Source: CAD feature listing. Evaluate the final solid. Frame: model axes, mm. A direction names the side the tool comes from. Round coordinates to 2 decimals unless told otherwise and drop trailing zeros. Loops run counter-clockwise (first coordinate to the right, second up) from the corner with the lowest first, then second, coordinate; pieces in that order, holes last.
Item 1: Access query for faces 5 (the flat face through (-18, 54.636, 13)), 6 (the cylindrical face through (-13.866, 9.46, 30.61)), 7 (the flat face through (-7, -33.534, 37)), 8 (the cylindrical face through (-19.275, 56.525, 38.298)). Directions: +Z, -Z, +X, -X, +Y, -Y. A direction counts if a zero-diameter tool reaches every point of the face in a straight line with its end or side. Return the directions, or none.
Item 2: Section query C-C on x = 0. Give the number of separate pieces and of enclosed holes in the cut face, then the cut area to 3 significant figures.
Item 3: First-contact query: P1, Ø8, axis at x = 31, z = 0, coming from the -Y side; P2, Ø1.2, axis at y = 72, z = 29.5, coming from the -X side; P3, Ø6, axis at x = -9, z = -20, coming from the -Y side; P4, Ø8, axis at x = -40, z = 63.97, coming from the +Y side. Flat tips, straight axial feed; report the tip coordinate or a pass-through.
Item 4: Ray query, L1, parallel to Z at x = -15, y = 20.5; L2, parallel to Y at x = 14, z = -9.5; L3, parallel to Y at x = -8, z = 33.5. Return the intervals inside material, ascending.
Item 5: Pull-direction query (Y, two-part tool) for faces 1 (the cylindrical face through (-53.16, -20.17, -12.46)), 2 (the cylindrical face through (-42.44, 117.75, -39.52)), 3 (the cylindrical face through (-13.866, 9.46, -5.616)), 4 (the cylindrical face through (-13.866, 9.46, -15.904)); classes: released by +Y, released by -Y, zero draft, split by the parting line, or undercut.
Item 6: Section query B-B on x = -55. Return loops of the section in (y, z), then the cut area to 3 significant figures.
```python
from build123d import *

# Parameters (mm, degrees)
SKETCH1_R                = 45
BOSS_EXTRUDE1_DEPTH      = 25
BOSS_EXTRUDE2_DEPTH      = 25
BOSS_EXTRUDE2_DEPTH_BACK = 60
SKETCH3_R                = 16.694420179
BOSS_EXTRUDE3_DEPTH      = 10
SKETCH4_W                = 70
SKETCH4_H                = 114.66
BOSS_EXTRUDE4_DEPTH      = 5
SKETCH5_R                = 16.667292011
BOSS_EXTRUDE5_DEPTH      = 14
BOSS_EXTRUDE5_DEPTH_BACK = 39
FILLET1_R                = 10
FILLET2_R                = 40
FILLET3_R                = 20
FILLET4_R                = 5
FILLET5_R                = 2
SCALE1_SCALE             = 1.111111111
SKETCH6_W                = 73.333333333
SKETCH6_H                = 122.955555555
BOSS_EXTRUDE6_DEPTH      = 90
SKETCH7_R                = 2.5
CUT_EXTRUDE1_DEPTH       = 239.92789275
CUT_EXTRUDE1_DEPTH_BACK  = 239.92789275


with BuildPart() as part:
    # Sketch1 → Boss-Extrude1 (new body)
    with BuildSketch(Plane.XY):
        Circle(SKETCH1_R)
    extrude(amount=BOSS_EXTRUDE1_DEPTH)



with BuildPart() as body_2:
    # Sketch2 → Boss-Extrude2 (new, two sides)
    with BuildSketch(Plane(origin=(0, 0, 0), x_dir=(0, 0, -1), z_dir=(1, 0, 0))) as boss_extrude2_sk:
        Polygon((-32.711176171, -28.552814356), (-32.711176171, 50.79995961), (7.711176171, 50.79995961), (7.711176171, -28.552814356), (12.147045523, -28.552814356), (12.147045523, 54.003643031), (-37.147045523, 54.003643031), (-37.147045523, -28.552814356), align=None)
    extrude(amount=BOSS_EXTRUDE2_DEPTH)
    extrude(boss_extrude2_sk.sketch, amount=-BOSS_EXTRUDE2_DEPTH_BACK)

    # Sketch3 → Boss-Extrude3 (add)
    with BuildSketch(Plane(origin=(0, 54.003643031, 0), x_dir=(1, 0, 0), z_dir=(0, 1, 0))):
        with Locations(Location((-20, -13.418920015, 0), (0, 0, 270))):
            Circle(SKETCH3_R)
    extrude(amount=BOSS_EXTRUDE3_DEPTH)

    # Sketch4 → Boss-Extrude4 (add)
    with BuildSketch(Plane(origin=(0, 64.003643031, 0), x_dir=(1, 0, 0), z_dir=(0, 1, 0))):
        with Locations((-20, -12.5)):
            Rectangle(SKETCH4_W, SKETCH4_H)
    extrude(amount=BOSS_EXTRUDE4_DEPTH)


with BuildPart() as part_1:
    add(part.part)

    add(body_2.part)  # Boss-Extrude5 merges body 2
    # Sketch5 → Boss-Extrude5 (add, two sides)
    with BuildSketch(Plane(origin=(0, 0, 0), x_dir=(-1, 0, 0), z_dir=(0, 0, -1))) as boss_extrude5_sk:
        with Locations(Location((0, 0, 0), (0, 0, 180))):
            Circle(SKETCH5_R)
    extrude(amount=BOSS_EXTRUDE5_DEPTH)
    extrude(boss_extrude5_sk.sketch, amount=-BOSS_EXTRUDE5_DEPTH_BACK)

    # Fillet1
    fillet1_edges = [part_1.edges().sort_by_distance(p)[0] for p in [
        (-45, 0, 0),
        (-45, 0, 25),
    ]]
    fillet(fillet1_edges, radius=FILLET1_R)

    # Fillet2
    fillet2_edges = [part_1.edges().sort_by_distance(p)[0] for p in [
        (-60, -28.552814356, 34.929110847),
        (-60, -28.552814356, -9.929110847),
    ]]
    fillet(fillet2_edges, radius=FILLET2_R)

    # Fillet3
    fillet3_edges = [part_1.edges().sort_by_distance(p)[0] for p in [
        (25, -28.552814356, 34.929110847),
        (25, -28.552814356, -9.929110847),
    ]]
    fillet(fillet3_edges, radius=FILLET3_R)

    # Fillet4
    fillet4_edges = [part_1.edges().sort_by_distance(p)[0] for p in [
        (-17.5, 54.003643031, 37.147045523),
        (-17.5, 54.003643031, -12.147045523),
        (-17.5, 50.79995961, -7.711176171),
        (-17.5, 50.79995961, 32.711176171),
    ]]
    fillet(fillet4_edges, radius=FILLET4_R)

    # Fillet5
    fillet5_edges = [part_1.edges().sort_by_distance(p)[0] for p in [
        (-55, 64.003643031, 12.5),
        (-20, 64.003643031, 69.83),
        (15, 64.003643031, 12.5),
        (-20, 64.003643031, -44.83),
        (-55, 69.003643031, 12.5),
        (-20, 69.003643031, 69.83),
        (15, 69.003643031, 12.5),
        (-20, 69.003643031, -44.83),
    ]]
    fillet(fillet5_edges, radius=FILLET5_R)


with BuildPart() as part_2:
    # Scale1: scaled about (-7.475087619, 16.274033837, 12.528539565)
    add(part_1.part.scale(SCALE1_SCALE).moved(Location((0.830565291, -1.808225982, -1.392059952))))


with BuildPart() as boss_extrude6_tool:
    # Sketch6 → Boss-Extrude6 (new body)
    with BuildSketch(Plane(origin=(0, 74.862466329, 0), x_dir=(1, 0, 0), z_dir=(0, 1, 0))):
        with Locations((-21.391645996, -12.49682915)):
            Rectangle(SKETCH6_W, SKETCH6_H)
    extrude(amount=BOSS_EXTRUDE6_DEPTH)


with BuildPart() as part_3:
    add(part_2.part)


with BuildPart() as part_4:
    # Boss-Extrude6: joined with boss_extrude6_tool
    add(part_3.part.fuse(boss_extrude6_tool.part, tol=0.00001))

    # Sketch7 → Cut-Extrude1 (cut, two sides)
    with BuildSketch(Plane(origin=(0, 164.862466329, 0), x_dir=(1, 0, 0), z_dir=(0, 1, 0))) as cut_extrude1_sk:
        with Locations(Location((0, 38.980948628, 0), (0, 0, 270))):
            Circle(SKETCH7_R)
        with Locations(Location((-40, 38.980948628, 0), (0, 0, 270))):
            Circle(SKETCH7_R)
        with Locations(Location((0, -63.974606927, 0), (0, 0, 270))):
            Circle(SKETCH7_R)
        with Locations(Location((-40, -63.974606927, 0), (0, 0, 270))):
            Circle(SKETCH7_R)
    extrude(amount=CUT_EXTRUDE1_DEPTH, mode=Mode.SUBTRACT)
    extrude(cut_extrude1_sk.sketch, amount=-CUT_EXTRUDE1_DEPTH_BACK, mode=Mode.SUBTRACT)


solid = part_4.part
```
Data:
1. face 5: +X, -X
1. face 6: none
1. face 7: +Z, +X, -X, -Y
1. face 8: +Z, +X, -X
2. separate pieces: 4
2. enclosed holes: 1
2. area: 15,300 mm2
3. P1: stops at y = -40.82
3. P2: stops at x = -60.28
3. P3: stops at y = 69.31
3. P4: stops at y = 164.86
4. L1: z = -14.89 to -9.96, -1.39 to 26.39, 34.95 to 39.88
4. L2: y = -14.83 to 11.21, 51.29 to 58.19, 69.31 to 164.86
4. L3: y = -18.09 to 14.47, 52.83 to 58.2, 69.31 to 164.86
5. face 1: released by -Y
5. face 2: zero draft
5. face 3: undercut
5. face 4: undercut
6. outline: (-18.17, -14.89) - (52.64, -14.89) arc R5.56 ccw to (58.2, -9.33) - (58.2, 34.33) arc R5.56 ccw to (52.64, 39.88) - (-18.17, 39.88) - (-18.17, 34.95) - (49.08, 34.95) arc R5.56 cw to (54.64, 29.4) - (54.64, -4.4) arc R5.56 cw to (49.08, -9.96) - (-18.17, -9.96) - close; (69.31, -48.98) arc R2.22 ccw to (71.53, -51.2) - (72.64, -51.2) arc R2.22 ccw to (74.86, -48.98) - (164.86, -48.98) - (164.86, 73.97) - (74.86, 73.97) arc R2.22 ccw to (72.64, 76.2) - (71.53, 76.2) arc R2.22 ccw to (69.31, 73.97) - close
6. area: 12,700 mm2
